The listing builds one solid part. Answer for the finished solid, in the listing's coordinates (mm). Face numbers are marked on the shaded views. Coordinates: 2 decimals unless noted, no trailing zeros. Write each loop counter-clockwise with the first axis right and the second up, starting at its lowest first coordinate (ties: lowest second). Pieces come first, ordered by that corner, then holes.
(1) The part is cut by section A-A on y = 51. Determine the outline of the cut face in (x, z).
(2) Given P1, Ø1.5, axis at x = 9, z = -35, coming from the +Y side; P2, Ø3, axis at x = -5.5, y = 26, coming from the +Z side; P3, Ø12, axis at x = -26, y = 74.5, coming from the +Z side; P4, Ø20.5, axis at x = 0, z = 0, coming from the -Y side, each flat-ended and moving along its own axis, determine where each tip first touches the part or whether it passes through.
(3) For a pull along Z with two mould halves and no side action, classify the marked faces 1, 2 and 3 as +Z half, -Z half, draft (parallel to the pull), parting line (faces both ways), or undercut.
(4) The part is cut by section B-B on y = 40. Determine the outline of the cut face in (x, z), plus the area to 3 significant figures.
(5) Straight lines are drawn through the part: line 1 (X direction, y = 66, z = 0) (3 decimals); line 2 (X direction, y = 44, z = 10); line 3 (Z direction, x = 12.5, y = 60.5). For each, find the intervals that lie inside material, in ascending order.
from build123d import *

# Parameters (mm, degrees)
SKETCH1_R            = 44.2849
BOSS_EXTRUDE1_DEPTH  = 86.106
FILLET1_R            = 2.54
MOVE_FACE1_OUTLINE_R = 44.2849
MOVE_FACE1_DEPTH     = 18.796


# Read off the part's stored shape, not the designer's step: Move Face1
with BuildPart() as part:
    # Sketch1 → Boss-Extrude1 (new body)
    with BuildSketch(Plane(origin=(0, 0, 0), x_dir=(1, 0, 0), z_dir=(0, 1, 0))):
        with Locations(Location((0, 0, 0), (0, 0, 270))):
            Circle(SKETCH1_R)
    extrude(amount=BOSS_EXTRUDE1_DEPTH)

    # Sketch2 → Cut-Revolve1 (revolve, cut)
    with BuildSketch(Plane.XY, mode=Mode.PRIVATE) as cut_revolve1_sk:
        Polygon((17.145, 70.358), (17.145, 62.738), (33.955596435, 0), (0, 0), (0, 86.106), (44.2849, 86.106), align=None)
    revolve(cut_revolve1_sk.sketch.rotate(Axis((0, 86.106, 0), (0, -1, 0)), 90), axis=Axis((0, 86.106, 0), (0, -1, 0)), mode=Mode.SUBTRACT)

    # Fillet1
    fillet1_edges = [part.edges().sort_by_distance(p)[0] for p in [
        (0, 70.358, -17.145),
        (0, 62.738, -17.145),
    ]]
    fillet(fillet1_edges, radius=FILLET1_R)

    # Move Face1 outline → Move Face1 (cut)
    with BuildSketch(Plane(origin=(0, 0, 0), x_dir=(1, 0, 0), z_dir=(0, 1, 0))):
        Circle(MOVE_FACE1_OUTLINE_R)
    extrude(amount=MOVE_FACE1_DEPTH, mode=Mode.SUBTRACT)


solid = part.part
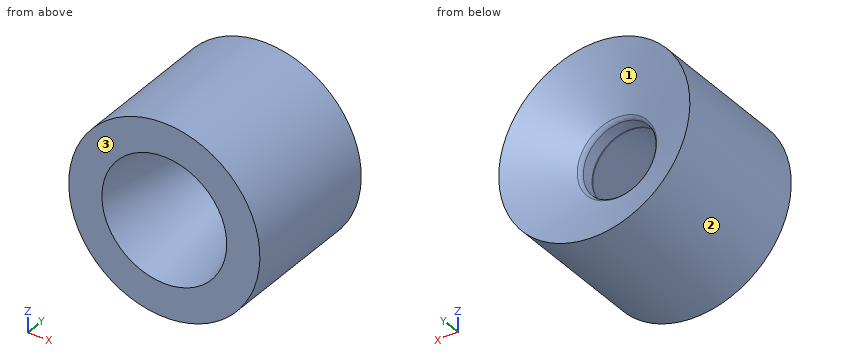
Model answer:
1. outline: circle Ø88.57 at (0, 0); hole circle Ø40.58 at (0, 0)
2. P1: stops at y = 81.81
2. P2: stops at z = 44.1
2. P3: stops at z = 39.51
2. P4: passes through
3. face 1: undercut
3. face 2: parting line
3. face 3: draft
4. outline: circle Ø88.57 at (0, 0); hole circle Ø46.48 at (0, 0)
4. area: 4,460 mm2
5. line 1: x = -44.285 to -17.145, 17.145 to 44.285
5. line 2: x = -43.14 to -19.78, 19.78 to 43.14
5. line 3: z = -42.48 to -12.59, 12.59 to 42.48
